Verification items for the finished model (mm, model axes). A direction names the side the tool comes from. Coordinates: 2 decimals unless noted, no trailing zeros. Loops run counter-clockwise (first coordinate to the right, second up) from the corner with the lowest first, then second, coordinate; pieces in that order, holes last. Notation, with made-up numbers: (10.5, -20) -> (51.5, -20) arc R21 cw to (51.5, 0) -> close; hole circle Ø5 at (-7.75, -14.75). An arc over 180 degrees is marked (long way). Write item = value, one per line.
Autodesk Inventor part; units mm, degrees
ref_plane "YZ Plane" through (0, 0, 0) normal (1, 0, 0) x (0, 1, 0)
ref_plane "XZ Plane" through (0, 0, 0) normal (0, 1, 0) x (-1, 0, 0)
ref_plane "XY Plane" through (0, 0, 0) normal (0, 0, 1) x (1, 0, 0)
sketch "Sketch1" plane through (0, 0, 0) normal (0, 0, 1) x (1, 0, 0)
  line L0 (0, 0) -> (0, -500) construction
  line L1 (0, 0) -> (6, 0)
  line L2 (6, 0) -> (6, -60)
  line L3 (6, -60) -> (9.2, -60)
  line L4 (9.2, -60) -> (9.2, -140)
  line L5 (9.2, -140) -> (6, -140)
  line L6 (6, -140) -> (6, -269.5)
  line L7 (0, 0) -> (0, -480)
  line L8 (0, 0) -> (0, 9) construction
  line L9 (4, -480) -> (4, -269.5)
  line L10 (4, -269.5) -> (6, -269.5)
  line L11 (4, -480) -> (0, -480)
  dimension "d1" = 12
  dimension "d2" = 60
  dimension "d3" = 18.4
  dimension "d4" = 80
  dimension "d7" = 8
  dimension "d8" = 210.5
  dimension "d9" = 480
revolve "Revolution1" add sketch "Sketch1" angle 360 about axis through (0, 0, 0) along (0, -1, 0)
sketch "Sketch2" plane through (0, -269.5, 0) normal (0, -1, 0) x (1, 0, 0)
  line L0 (0, 0) -> (0, 10.7217) construction
  line L1 (0, 0) -> (0, -10) construction
  line L2 (0, 0) -> (-12.4689, 0) construction
  line L3 (0, 0) -> (11.6918, 0) construction
  circle A0 centre (0, 0) radius 6 construction
  arc A1 (6, 0) -> (0, 6) centre (0, 0) ccw
  arc A2 (-6, 0) -> (0, -6) centre (0, 0) ccw
  arc A3 (4, 0) -> (0, 4) centre (0, 0) ccw
  arc A4 (-4, 0) -> (0, -4) centre (0, 0) ccw
  line L4 (-4, 0) -> (-6, 0)
  line L5 (0, -4) -> (0, -6)
  line L6 (0, 4) -> (0, 6)
  line L7 (4, 0) -> (6, 0)
  dimension "d10" = 4
  dimension "d11" = 4
extrude "Extrusion1" add sketch "Sketch2" along normal blind 5
sketch "Sketch3" plane through (0, -480, 0) normal (0, -1, 0) x (1, 0, 0)
  point P0 (0, 0)
  point P1 (0, 0)
hole "Hole1" at (0, -480, 0) direction (0, 1, 0) diameter 1.567 depth 6.3 tip angle 118
sketch "Sketch4" plane through (0, -480, 0) normal (0, -1, 0) x (1, 0, 0)
  point P0 (0, 0)
sketch "Sketch6" plane through (0, -480, 0) normal (0, -1, 0) x (1, 0, 0)
  point P0 (0, 0)
properties part number "Achse"
1) Sectioned sample at A-A, the plane y = -64. Record the cut outline in (x, z), plus the area to 3 significant figures.
Ans:
outline = circle Ø18.4 at (0, 0)
area = 266 mm2
2) Material ranges on line 1 (X direction, y = -476.5, z = 0); line 2 (Y direction, x = 4, z = 6.75), recorded low to high.
Ans:
line_1 = -4 to -0.78, 0.78 to 4
line_2 = -140 to -60
3) Depth check by flat-ended pin: pin 1 Ø0.6 at (y, z) = (-273, 5) entering from -X; pin 2 Ø5.5 at (x, z) = (-3, 4) entering from +Y; pin 3 Ø1 at (x, y) = (-5, -272.5) entering from +Z; pin 4 Ø3 at (x, z) = (-7, -4.5) entering from -Y. Enter the tip coordinate at first touch or a pass-through.
Ans:
pin_1 = 0
pin_2 = 0
pin_3 = 0
pin_4 = -140
4) Sectioned sample at B-B, the plane y = -424.5. Record the cut outline in (x, z), plus the area to 3 significant figures.
Ans:
outline = circle Ø8 at (0, 0)
area = 50.3 mm2
5) Tool access check on faces 1 (the face through (0, 0, 0)), 2 (the face through (-6, -30, 0)), 3 (the face through (-6, -208, 0)). Record the directions out of +Z, -Z, +X, -X, +Y, -Y that give a thin tool (end or side, any length) a straight path to the whole face; none if there is none.
Ans:
face_1 = +Z, -Z, +X, -X, +Y
face_2 = +Y
face_3 = -Y
